The listing builds one solid part. Answer for the finished solid, in the listing's coordinates (mm). A direction names the side the tool comes from. Coordinates: 2 decimals unless noted, no trailing zeros. Order: outer loops, then holes, each group sorted by start corner. A loop starts at its lowest first (then second) coordinate and runs counter-clockwise, first axis right, second up. Notation, with made-up numbers: (21.25, -5.5) -> (67.25, -5.5) arc R14 ccw to (67.25, -1.5) -> close; hole circle Ø9 at (-17.5, 6.25). An arc over 180 degrees is marked (long way). Write each question's results on one line, items separated by ' | '. Start each with the question number.
(1) Given pin 1 (4 mm diameter, centred on x = 15, z = 10, fed in from +Y); pin 2 (1 mm diameter, centred on y = 17, z = 2, fed in from -X); pin 3 (1.1 mm diameter, centred on y = 8.5, z = -0.5, fed in from +X), each flat-ended and moving along its own axis, determine where each tip first touches the part or whether it passes through.
(2) The part is cut by section A-A, the plane x = 15. Give the vertices of the cut face in (y, z), then the cut area to 3 significant figures.
(3) Straight lines are drawn through the part: L1, parallel to Y at x = 7.25, z = 2.5; L2, parallel to X at y = -1.3, z = 9; L3, parallel to X at y = -0.75, z = 10. For each, find the intervals that lie inside material, in ascending order.
(4) The part is cut by section D-D, the plane y = 7. Give the vertices of the cut face in (x, z), then the cut area to 3 significant figures.
(5) The part is cut by section B-B, the plane z = 7. Give the vertices of the cut face in (x, y).
(6) A tool of negligible diameter and unlimited length cuts with its end or side. For faces 1 (the face through (16.39, -1.01, 9.11)), 2 (the face through (15, 18, 19)), 3 (the face through (28.11, 8.77, -0.99)), 4 (the face through (15, 9, 0)), 5 (the face through (21.75, 8, -1)), from which of +Z, -Z, +X, -X, +Y, -Y can it reach the whole face along a straight path? Write none if from no direction.
(7) The part is cut by section C-C, the plane x = 3.25. Give the vertices of the cut face in (y, z), then the cut area to 3 significant figures.
(8) Determine the mould class of faces 6 (the face through (25.75, 8, -1)), 7 (the face through (24.206, 14.606, -1.014)), 8 (the face through (3.137, -0.986, 15.692)) for opening direction X: +X half, -X half, draft (parallel to the pull), parting line (faces both ways), or undercut.
```python
from build123d import *

# Parameters (mm, degrees)
BRIDA_BASE1_DEPTH                = 2
REDONDEO3MM_R                    = 3
BRIDA_DE_ARISTA1_STRIP_W         = 10
BRIDA_DE_ARISTA1_STRIP_H         = 2
BRIDA_DE_ARISTA1_STRIP_CUT_DEPTH = 30
BRIDA_DE_ARISTA1_DEPTH           = 30
BRIDA_DE_ARISTA2_STRIP_W         = 10
BRIDA_DE_ARISTA2_STRIP_H         = 2
BRIDA_DE_ARISTA2_STRIP_CUT_DEPTH = 18
BRIDA_DE_ARISTA2_DEPTH           = 18
BRIDA_START                      = 2
BRIDA_DE_ARISTA2_FLAT_DEPTH      = 2
CORTAR_EXTRUIR6_REACH            = 43.255
REDONDEO11MM_R                   = 11
TALADRO_ROSCADO_M32_D            = 2.5
TALADRO_ROSCADO_M32_DEPTH        = 20.65
TALADRO_ROSCADO_M32_TIP          = 0.751075774
CROQUIS41_R                      = 2.05
CORTAR_EXTRUIR9_DEPTH            = 2
TALADRO_ROSCADO_M41_D            = 3.3


# Sheet-metal steps are written as plain solids
with BuildPart() as part:
    # Croquis1 → Brida base1 (new body)
    with BuildSketch(Plane.XY):
        with BuildLine():
            Line((0, 0), (30, 0))
            Line((30, 0), (30, 3))
            ThreePointArc((30, 3), (27.886584846, 9.212566007), (24, 14.5))
            Line((24, 14.5), (24, 17))
            Line((24, 17), (6, 17))
            Line((6, 17), (6, 14.5))
            ThreePointArc((6, 14.5), (2.113415154, 9.212566007), (0, 3))
            Line((0, 3), (0, 0))
        make_face()
    extrude(amount=-BRIDA_BASE1_DEPTH)

    # Redondeo3mm
    redondeo3mm_edges = [part.edges().sort_by_distance(p)[0] for p in [
        (0, 3, -1),
        (6, 14.5, -1),
        (24, 14.5, -1),
        (30, 3, -1),
    ]]
    fillet(redondeo3mm_edges, radius=REDONDEO3MM_R)

    # Brida de arista1 strip (across the edge) → Brida de arista1 strip cut (cut)
    with BuildSketch(Plane.YZ):
        with Locations((-4, -1)):
            Rectangle(BRIDA_DE_ARISTA1_STRIP_W, BRIDA_DE_ARISTA1_STRIP_H)
    extrude(amount=BRIDA_DE_ARISTA1_STRIP_CUT_DEPTH, mode=Mode.SUBTRACT)

    # Brida de arista1 section (across the edge) → Brida de arista1 (add)
    with BuildSketch(Plane.YZ):
        with BuildLine():
            Line((-2, 1), (-2, 19))
            Line((-2, 19), (0, 19))
            Line((0, 19), (0, 1))
            ThreePointArc((0, 1), (0.292893219, 0.292893219), (1, 0))
            Line((1, 0), (1, -2))
            ThreePointArc((1, -2), (-1.121320344, -1.121320344), (-2, 1))
        make_face()
    extrude(amount=BRIDA_DE_ARISTA1_DEPTH)

    # Brida de arista2 strip (across the edge) → Brida de arista2 strip cut (cut)
    with BuildSketch(Plane(origin=(24, 17, 0), x_dir=(0, -1, 0), z_dir=(-1, 0, 0))):
        with Locations((-4, -1)):
            Rectangle(BRIDA_DE_ARISTA2_STRIP_W, BRIDA_DE_ARISTA2_STRIP_H)
    extrude(amount=BRIDA_DE_ARISTA2_STRIP_CUT_DEPTH, mode=Mode.SUBTRACT)

    # Brida de arista2 bend section (across the edge) → Brida de arista2 (add)
    with BuildSketch(Plane(origin=(24, 17, 0), x_dir=(0, -1, 0), z_dir=(-1, 0, 0))):
        with BuildLine():
            Line((-2, 1), (0, 1))
            ThreePointArc((0, 1), (0.292893219, 0.292893219), (1, 0))
            Line((1, 0), (1, -2))
            ThreePointArc((1, -2), (-1.121320344, -1.121320344), (-2, 1))
        make_face()
    extrude(amount=BRIDA_DE_ARISTA2_DEPTH)

    # Brida de arista2 profile (on flange) → Brida de arista2 flat (add)
    with BuildSketch(Plane(origin=(0, 17, 0), x_dir=(-1, 0, 0), z_dir=(0, 1, 0)).offset(BRIDA_START)):
        with BuildLine():
            ThreePointArc((-6, 10), (-15, 19), (-24, 10))
            Line((-24, 10), (-24, 1))
            Line((-24, 1), (-6, 1))
            Line((-6, 1), (-6, 10))
        make_face()
    extrude(amount=-BRIDA_DE_ARISTA2_FLAT_DEPTH)

    # Croquis26 → Cortar-Extruir6 (cut, up to next)
    with BuildSketch(Plane(origin=(0, 0, -2), x_dir=(-1, 0, 0), z_dir=(0, 0, -1)), mode=Mode.PRIVATE) as cortar_extruir6_sk1:
        with BuildLine():
            Line((-8.25, 7.8), (-8.25, 8.8))
            ThreePointArc((-8.25, 8.8), (-6.25, 10.8), (-4.25, 8.8))
            Line((-4.25, 8.8), (-4.25, 7.8))
            ThreePointArc((-4.25, 7.8), (-6.25, 5.8), (-8.25, 7.8))
        make_face()
    cortar_extruir6_tool1 = extrude(cortar_extruir6_sk1.sketch, amount=-CORTAR_EXTRUIR6_REACH, mode=Mode.PRIVATE) & part.part
    # Croquis26 → Cortar-Extruir6 (cut, up to next)
    with BuildSketch(Plane(origin=(0, 0, -2), x_dir=(-1, 0, 0), z_dir=(0, 0, -1)), mode=Mode.PRIVATE) as cortar_extruir6_sk2:
        with BuildLine():
            Line((-25.75, 7.8), (-25.75, 8.8))
            ThreePointArc((-25.75, 8.8), (-23.75, 10.8), (-21.75, 8.8))
            Line((-21.75, 8.8), (-21.75, 7.8))
            ThreePointArc((-21.75, 7.8), (-23.75, 5.8), (-25.75, 7.8))
        make_face()
    cortar_extruir6_tool2 = extrude(cortar_extruir6_sk2.sketch, amount=-CORTAR_EXTRUIR6_REACH, mode=Mode.PRIVATE) & part.part
    add(cortar_extruir6_tool1.solids().sort_by_distance((6.25, 8.3, -2))[0], mode=Mode.SUBTRACT)
    add(cortar_extruir6_tool2.solids().sort_by_distance((23.75, 8.3, -2))[0], mode=Mode.SUBTRACT)

    # Redondeo11mm
    redondeo11mm_edges = [part.edges().sort_by_distance(p)[0] for p in [
        (0, -1, 19),
        (30, -1, 19),
    ]]
    fillet(redondeo11mm_edges, radius=REDONDEO11MM_R)

    # Taladro roscado M32
    with Locations(Plane(origin=(0, 0, 0), x_dir=(1, 0, 0), z_dir=(0, 1, 0))):
        with Locations((3.25, -9), (26.75, -9)):
            Hole(TALADRO_ROSCADO_M32_D / 2, depth=TALADRO_ROSCADO_M32_DEPTH)
            with Locations((0, 0, -(TALADRO_ROSCADO_M32_DEPTH + TALADRO_ROSCADO_M32_TIP / 2))):  # 118° drill point
                Cone(0, TALADRO_ROSCADO_M32_D / 2, TALADRO_ROSCADO_M32_TIP, mode=Mode.SUBTRACT)

    # Croquis41 → Cortar-Extruir9 (cut)
    with BuildSketch(Plane(origin=(0, 19, 0), x_dir=(1, 0, 0), z_dir=(0, 1, 0))):
        with Locations(Location((15, -10, 0), (0, 0, 270))):
            Circle(CROQUIS41_R)
    extrude(amount=-CORTAR_EXTRUIR9_DEPTH, mode=Mode.SUBTRACT)

    # Taladro roscado M41 (through all)
    with Locations(Plane(origin=(15, 0, 10), x_dir=(0, 0, 1), z_dir=(0, 1, 0))):
        with Locations((0, 0)):
            Hole(TALADRO_ROSCADO_M41_D / 2)


solid = part.part
```
Established:
1) pin 1: stops at y = 0 | pin 2: stops at x = 6 | pin 3: stops at x = 28.49
2) outline: (-2, 1) arc R3 ccw to (1, -2) -> (16, -2) arc R3 ccw to (19, 1) -> (19, 7.95) -> (17, 7.95) -> (17, 1) arc R1 cw to (16, 0) -> (1, 0) arc R1 cw to (0, 1) -> (0, 8.35) -> (-2, 8.35) -> close; (-2, 11.65) -> (0, 11.65) -> (0, 19) -> (-2, 19) -> close; (17, 12.05) -> (19, 12.05) -> (19, 19) -> (17, 19) -> close | area: 99.8 mm^2
3) L1: y = -2 to 0, 17 to 19 | L2: x = 0.05 to 2, 4.5 to 13.69, 16.31 to 25.5, 28 to 29.95 | L3: x = 0.18 to 2.5, 4 to 13.35, 16.65 to 26, 27.5 to 29.82
4) outline: (1.11, -2) -> (4.42, -2) -> (4.42, 0) -> (1.11, 0) -> close; (8.08, -2) -> (21.92, -2) -> (21.92, 0) -> (8.08, 0) -> close; (25.58, -2) -> (28.89, -2) -> (28.89, 0) -> (25.58, 0) -> close | area: 40.9 mm^2
5) outline: (0, -2) -> (30, -2) -> (30, 0) -> (0, 0) -> close; (6, 17) -> (24, 17) -> (24, 19) -> (6, 19) -> close
6) face 1: +Y, -Y | face 2: +Z, +Y | face 3: +Z, -Z, +X, +Y | face 4: +Z, +X, -X | face 5: +Z, -Z
7) outline: (-2, 1) arc R3 ccw to (1, -2) -> (11.14, -2) -> (11.14, 0) -> (1, 0) arc R1 cw to (0, 1) -> (0, 7.75) -> (-2, 7.75) -> close; (-2, 10.25) -> (0, 10.25) -> (0, 15.81) -> (-2, 15.81) -> close | area: 51.2 mm^2
8) face 6: undercut | face 7: +X half | face 8: -X half
